from build123d import *

# Parameters (mm, degrees)
BOSS_EXTRUDE1_DEPTH = 5


with BuildPart() as part:
    # Sketch1 → Boss-Extrude1 (new body)
    with BuildSketch(Plane(origin=(0, 0, 0), x_dir=(1, 0, 0), z_dir=(0, 1, 0))):
        with BuildLine():
            Line((-457.208642176, 422.631578947), (-351.296475424, 422.631578947))
            Line((-351.296475424, 422.631578947), (-351.296475424, 222.631578947))
            Line((-351.296475424, 222.631578947), (-457.208642176, 222.631578947))
            Line((-457.208642176, 222.631578947), (-457.208642176, 121.631578947))
            ThreePointArc((-457.208642176, 121.631578947), (-460.137574364, 114.560511136), (-467.208642176, 111.631578947))
            Line((-467.208642176, 111.631578947), (-472.208642176, 111.631578947))
            ThreePointArc((-472.208642176, 111.631578947), (-479.279709988, 114.560511136), (-482.208642176, 121.631578947))
            Line((-482.208642176, 121.631578947), (-482.208642176, 222.631578947))
            Line((-482.208642176, 222.631578947), (-691.296475424, 222.631578947))
            Line((-691.296475424, 222.631578947), (-691.296475424, 422.631578947))
            Line((-691.296475424, 422.631578947), (-482.208642176, 422.631578947))
            Line((-482.208642176, 422.631578947), (-482.208642176, 523.631578947))
            ThreePointArc((-482.208642176, 523.631578947), (-479.279709988, 530.702646759), (-472.208642176, 533.631578947))
            Line((-472.208642176, 533.631578947), (-467.208642176, 533.631578947))
            ThreePointArc((-467.208642176, 533.631578947), (-460.137574364, 530.702646759), (-457.208642176, 523.631578947))
            Line((-457.208642176, 523.631578947), (-457.208642176, 422.631578947))
        make_face()
    extrude(amount=BOSS_EXTRUDE1_DEPTH)


solid = part.part
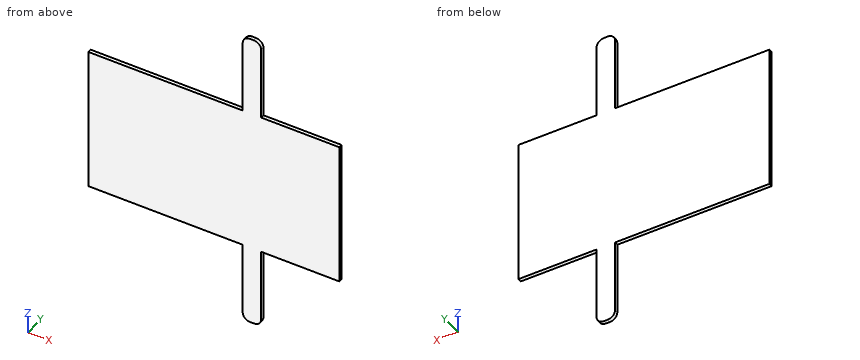
Could you check a few things on this model? Use its own coordinates, in mm. Give positions to 0.01 mm unless a question says otherwise; leave off trailing zeros. Loops run counter-clockwise (first coordinate to the right, second up) from the corner with the lowest first, then second, coordinate; pieces in that order, holes last. Notation, with made-up numbers: M 1,-32.75 L 49,-32.75 A6 cw 49,-21.75 Z; hole C -14.75,60 d3. An arc over 180 degrees is marked long. Answer as a JSON object with one key per item and string values.
Q1. Suppose I cut it at B-B, the plane z = -427. List the corners of the cut face in (x, y) for me, plus the area to 3 significant figures.
Values found:
{"outline": "M -482.21,0 L -457.21,0 L -457.21,5 L -482.21,5 Z", "area": "125 mm²"}
Q2. Suppose I cut it at C-C, the plane x = -538. List the corners of the cut face in (y, z) for me, plus the area to 3 significant figures.
Values found:
{"outline": "M 0,-422.63 L 5,-422.63 L 5,-222.63 L 0,-222.63 Z", "area": "1,000 mm²"}
Q3. For P1, Ø1, axis at x = -417, y = 1.5, coming from the +Z side, with a flat end and sliding along its axis, tell me the tip position at first contact or that it passes through.
Values found:
{"P1": "stops at z = -222.63"}
Q4. Suppose I cut it at A-A, the plane y = 2.1. List the corners of the cut face in (x, z) for me, plus the area to 3 significant figures.
Values found:
{"outline": "M -691.3,-422.63 L -482.21,-422.63 L -482.21,-523.63 A10 ccw -472.21,-533.63 L -467.21,-533.63 A10 ccw -457.21,-523.63 L -457.21,-422.63 L -351.3,-422.63 L -351.3,-222.63 L -457.21,-222.63 L -457.21,-121.63 A10 ccw -467.21,-111.63 L -472.21,-111.63 A10 ccw -482.21,-121.63 L -482.21,-222.63 L -691.3,-222.63 Z", "area": "73,500 mm²"}
Q5. If I drill on probe 1 along Z at (x, y) = (-569.5, 0.7); probe 2 along X at (y, z) = (4.7, -426); probe 3 along Z at (x, y) = (-481, 2.6), over which ranges is the centre line in solid material (lowest first)? Write a range as [from, to].
Values found:
{"probe 1": "z = [-422.63, -222.63]", "probe 2": "x = [-482.21, -457.21]", "probe 3": "z = [-528.4, -116.87]"}
